Geometry: see drawing. Coordinates: mm, zero at the bounding-box minimum. A direction names the side the tool comes from. Give positions to 0.01 mm unless a question says otherwise; leave off trailing zeros. Order: outer loops, then holes, each group sorted by start corner. A loop starts at its lowest first (then second) coordinate and runs counter-clockwise, first axis right, second up. Notation, with made-up numbers: M 72,46 L 105,46 A30 ccw 105,73 Z; hole C 62,-20 d3. An arc over 180 degrees is marked long. Answer as a JSON object with one key per item and string values. Group by question number.
1. Section query B-B (y = 3). Output: boundary loops of the cut face in (x, z), plus the area to 3 significant figures.
2. Section query D-D (z = 9). Count the separate pieces of the cut face and the enclosed holes in it, plus the area to 3 significant figures.
3. Set-up query: the marked faces 5, 6 and 7. Return all of +Z, -Z, +X, -X, +Y, -Y with unobstructed straight access to the full face (end or side cutting, diameter ignored); none if empty.
4. Material intervals for L1, parallel to X at y = 4.5, z = 9.25; L2, parallel to Z at x = 36, y = 5.75; L3, parallel to X at y = 3.75, z = 10, sorted ascending. Write a range as [from, to].
5. Section query A-A (x = 6). Output: boundary loops of the cut face in (y, z).
6. Pull-direction query (Y, two-part tool) for the marked faces 1, 2, 3 and 4; classes: +Y half, -Y half, draft (parallel to the pull), parting line (faces both ways), or undercut.
7. Pin query (flat end, axial travel): P1, Ø6, axis at x = 7, z = 5.5, coming from the -Y side; P2, Ø5.5, axis at x = 36, z = 9, coming from the -Y side; P3, Ø6, axis at x = 34, z = 9.5, coming from the +Y side; P4, Ø2.5, axis at y = 13, z = 5, coming from the +X side. Return the tip coordinate at first contact, or that it passes through.
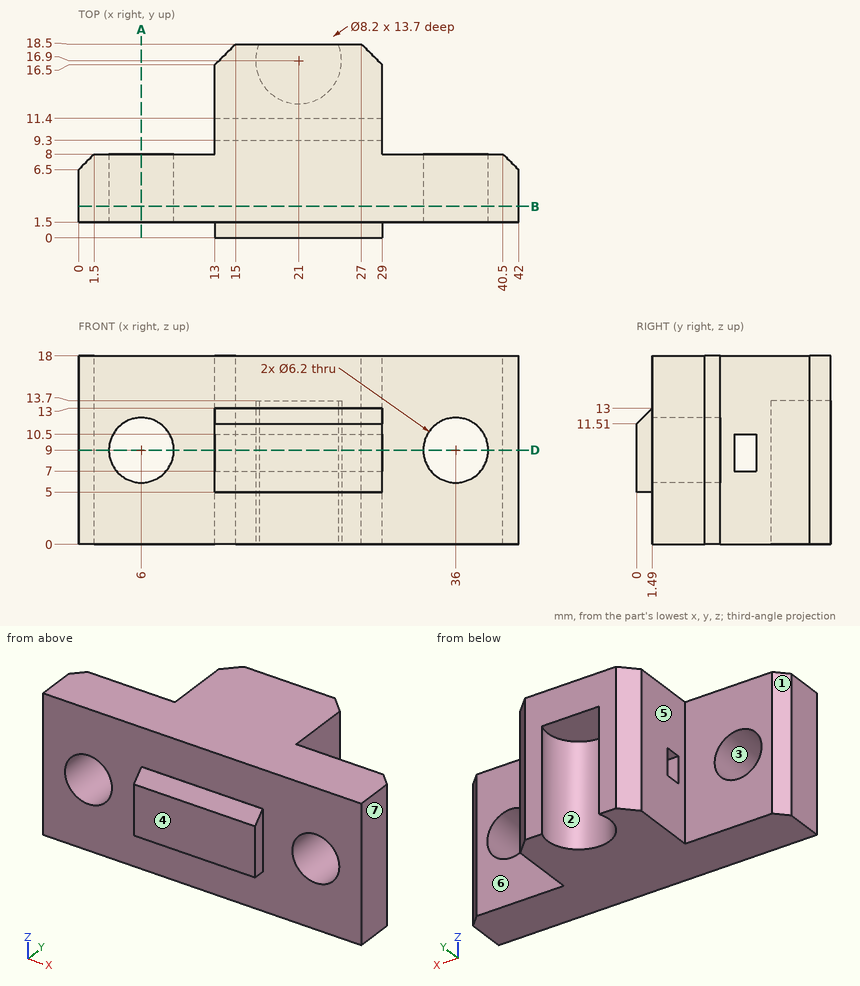
Answer sheet:
{
 "1": {"outline": "M 0,0 L 42,0 L 42,18 L 0,18 Z; hole C 6,9 d6.2; hole C 36,9 d6.2", "area": "696 mm^2"},
 "2": {"separate pieces": "4", "enclosed holes": "0", "area": "305 mm^2"},
 "3": {"face 5": "+Z, -Z, -X, +Y", "face 6": "+Z, -Z, +X, +Y", "face 7": "+Z, -Z, +X, +Y, -Y"},
 "4": {"L1": "[0, 2.91], [9.09, 32.91], [39.09, 42]", "L2": "[0, 5.9], [12.1, 18]", "L3": "[0, 3.07], [8.93, 33.07], [38.93, 42]"},
 "5": {"outline": "M 1.5,0 L 8,0 L 8,5.9 L 1.5,5.9 Z; M 1.5,12.1 L 8,12.1 L 8,18 L 1.5,18 Z"},
 "6": {"face 1": "+Y half", "face 2": "undercut", "face 3": "draft", "face 4": "-Y half"},
 "7": {"P1": "y = 1.5", "P2": "through", "P3": "y = 8", "P4": "x = 29"}
}
